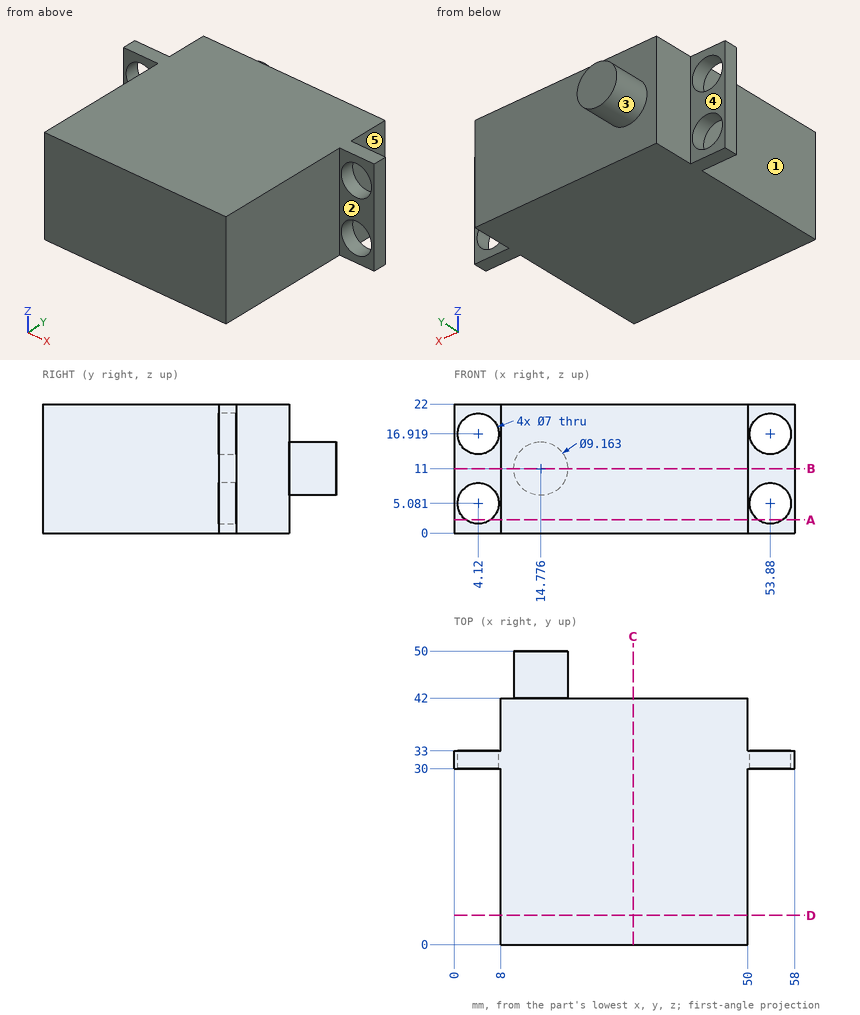
Design review of the part shown in the three views and the two pictorial views. Dimensions are in mm from the part's minimum x, y and z. A direction names the side the tool comes from. Coordinates: 2 decimals unless noted, no trailing zeros. Loops run counter-clockwise (first coordinate to the right, second up) from the corner with the lowest first, then second, coordinate; pieces in that order, holes last.
(1) Consider section C-C, the plane x = 30.5. Give the boundary of the cut face in (y, z), plus the area to 3 significant figures.
Determined:
outline: (0, 0) - (42, 0) - (42, 22) - (0, 22) - close
area: 924 mm2
(2) Consider section B-B, the plane z = 11. Give the boundary of the cut face in (x, y) (1 decimal), plus the area to 3 significant figures.
Determined:
outline: (0, 30) - (8, 30) - (8, 0) - (50, 0) - (50, 30) - (58, 30) - (58, 33) - (50, 33) - (50, 42) - (19.4, 42) - (19.4, 50) - (10.2, 50) - (10.2, 42) - (8, 42) - (8, 33) - (0, 33) - close
area: 1,890 mm2
(3) Wall thickness on L1, parallel to X at y = 23.5, z = 3; L2, parallel to Y at x = 24, z = 16.25; L3, parallel to X at y = 31.5, z = 18: over which ranges is each line inside the solid? List them lowest first.
Determined:
L1: x = 8 to 50
L2: y = 0 to 42
L3: x = 0 to 0.79, 7.45 to 50.55, 57.21 to 58
(4) Insertion check: P1, Ø4, axis at x = 4.12, z = 5.08, coming from the +Y side; P2, Ø4, axis at y = 36.5, z = 16, coming from the +X side; P3, Ø10, axis at y = 39.5, z = 13, coming from the -X side; P4, Ø4, axis at x = 2.5, z = 7.5, coming from the -Y side. Each pin has a flat end and moves straight along its axis. Give the tip position at first contact, or say it passes through.
Determined:
P1: passes through
P2: stops at x = 50
P3: stops at x = 8
P4: stops at y = 30
(5) Consider section A-A, the plane z = 2.25. Give the boundary of the cut face in (x, y), plus the area to 3 significant figures.
Determined:
outline: (0, 30) - (2.06, 30) - (2.06, 33) - (0, 33) - close; (6.18, 30) - (8, 30) - (8, 0) - (50, 0) - (50, 30) - (51.82, 30) - (51.82, 33) - (50, 33) - (50, 42) - (8, 42) - (8, 33) - (6.18, 33) - close; (55.94, 30) - (58, 30) - (58, 33) - (55.94, 33) - close
area: 1,790 mm2
(6) Consider section D-D, the plane y = 5. Give the boundary of the cut face in (x, z).
Determined:
outline: (8, 0) - (50, 0) - (50, 22) - (8, 22) - close
(7) Tool access review of the marked faces 1, 2, 3, 4 and 5: name each direction out of +Z, -Z, +X, -X, +Y, -Y from which nothing blocks a thin tool from reaching the whole face with its end or side.
Determined:
face 1: +Z, -Z, -X, -Y
face 2: +Z, -Z, +X, -Y
face 3: +Y
face 4: +Z, -Z, -X, +Y
face 5: +Z, -Z, +X, +Y
